Could you check a few things on this model? Use its own coordinates, in mm. A direction names the side the tool comes from. Give positions to 0.01 mm unless a question says otherwise; leave off trailing zeros. Loops run counter-clockwise (first coordinate to the right, second up) from the corner with the lowest first, then second, coordinate; pieces in that order, holes last. Notation, with made-up numbers: (32.25, 50.5) -> (47.25, 50.5) arc R17 ccw to (47.25, 75.5) -> close; hole circle Ø4 at (7.5, 70.5). An arc over 180 degrees is marked (long way). Put each result on its own line as item: value.
```python
from build123d import *

# Parameters (mm, degrees)
SKETCH1_R             = 25
BOSS_EXTRUDE1_DEPTH   = 12.38
BOSS_EXTRUDE4_START   = -5.38
SKETCH9_R             = 25
SKETCH9_R_2           = 9.525
BOSS_EXTRUDE4_DEPTH   = 5.38
SKETCH4_OUTSIDE_W     = 66.358
SKETCH4_OUTSIDE_H     = 66.358
SKETCH4_OUTSIDE_R     = 22
TREAD_CLEARANCE_DEPTH = 38.460170849
CUT_EXTRUDE2_START    = 1
SKETCH5_OUTSIDE_W     = 58.688
SKETCH5_OUTSIDE_H     = 58.688
SKETCH5_OUTSIDE_R     = 21.7
CUT_EXTRUDE2_DEPTH    = 10.38
CUT_EXTRUDE3_DEPTH    = 10.38
CIRPATTERN4_COUNT     = 18


with BuildPart() as part:
    # Sketch1 → Boss-Extrude1 (new body)
    with BuildSketch(Plane.XY):
        with Locations(Location((0, 0, 0), (0, 0, 90))):
            Circle(SKETCH1_R)
        with BuildLine():
            Line((9.525, -7.110786438), (9.525, 7.110786438))
            ThreePointArc((9.525, 7.110786438), (9.448879533, 7.49346987), (9.232106781, 7.817893219))
            Line((9.232106781, 7.817893219), (7.817893219, 9.232106781))
            ThreePointArc((7.817893219, 9.232106781), (7.49346987, 9.448879533), (7.110786438, 9.525))
            Line((7.110786438, 9.525), (-7.110786438, 9.525))
            ThreePointArc((-7.110786438, 9.525), (-7.49346987, 9.448879533), (-7.817893219, 9.232106781))
            Line((-7.817893219, 9.232106781), (-9.232106781, 7.817893219))
            ThreePointArc((-9.232106781, 7.817893219), (-9.448879533, 7.49346987), (-9.525, 7.110786438))
            Line((-9.525, 7.110786438), (-9.525, -7.110786438))
            ThreePointArc((-9.525, -7.110786438), (-9.448879533, -7.49346987), (-9.232106781, -7.817893219))
            Line((-9.232106781, -7.817893219), (-7.817893219, -9.232106781))
            ThreePointArc((-7.817893219, -9.232106781), (-7.49346987, -9.448879533), (-7.110786438, -9.525))
            Line((-7.110786438, -9.525), (7.110786438, -9.525))
            ThreePointArc((7.110786438, -9.525), (7.49346987, -9.448879533), (7.817893219, -9.232106781))
            Line((7.817893219, -9.232106781), (9.232106781, -7.817893219))
            ThreePointArc((9.232106781, -7.817893219), (9.448879533, -7.49346987), (9.525, -7.110786438))
        make_face(mode=Mode.SUBTRACT)
    extrude(amount=BOSS_EXTRUDE1_DEPTH)

    # Sketch9 → Boss-Extrude4 (add)
    with BuildSketch(Plane.XY.offset(12.38).offset(BOSS_EXTRUDE4_START)):
        with Locations(Location((0, 0, 0), (0, 0, 90))):
            Circle(SKETCH9_R)
        Circle(SKETCH9_R_2, mode=Mode.SUBTRACT)
    extrude(amount=BOSS_EXTRUDE4_DEPTH)

    # Sketch4 outside → Tread Clearance (cut, through all)
    with BuildSketch(Plane.XY.offset(12.38)):
        Rectangle(SKETCH4_OUTSIDE_W, SKETCH4_OUTSIDE_H)
        Circle(SKETCH4_OUTSIDE_R, mode=Mode.SUBTRACT)
    extrude(amount=-TREAD_CLEARANCE_DEPTH, mode=Mode.SUBTRACT)

    # Sketch5 outside → Cut-Extrude2 (cut)
    with BuildSketch(Plane.XY.offset(CUT_EXTRUDE2_START)):
        Rectangle(SKETCH5_OUTSIDE_W, SKETCH5_OUTSIDE_H)
        with Locations(Location((0, 0, 0), (0, 0, 90))):
            Circle(SKETCH5_OUTSIDE_R, mode=Mode.SUBTRACT)
    extrude(amount=CUT_EXTRUDE2_DEPTH, mode=Mode.SUBTRACT)

    # Sketch6 → Cut-Extrude3 (cut)
    with BuildSketch(Plane.XY.offset(1)):
        with BuildLine():
            ThreePointArc((6.505756366, 20.361958768), (6.446827822, 19.666593295), (6.273572546, 18.99058418))
            ThreePointArc((6.273572546, 18.99058418), (6.465736016, 18.325211027), (7.157089189, 18.284235134))
            ThreePointArc((7.157089189, 18.284235134), (8.371042068, 18.936944495), (9.657089189, 19.432720561))
            ThreePointArc((9.657089189, 19.432720561), (8.132554572, 20.118438213), (6.559758729, 20.684766506))
            ThreePointArc((6.559758729, 20.684766506), (6.519461312, 20.525586959), (6.505756366, 20.361958768))
        make_face()
    cut_extrude3 = extrude(amount=CUT_EXTRUDE3_DEPTH, mode=Mode.SUBTRACT)

    # CirPattern4: Cut-Extrude3 ×18 about axis
    cirpattern4_axis = Axis((0, 0, 0), (0, 0, 1))
    for i in range(1, CIRPATTERN4_COUNT):
        add(cut_extrude3.rotate(cirpattern4_axis, i * 360 / CIRPATTERN4_COUNT), mode=Mode.SUBTRACT)


solid = part.part
```
1. I'm going to push flat-ended pins straight in: pin 1 (5 mm diameter, centred on y = 13, z = 1.5, fed in from -X); pin 2 (2 mm diameter, centred on x = -3.5, z = 10.5, fed in from -Y); pin 3 (2 mm diameter, centred on y = -0.5, z = 7, fed in from -X). Where does each tip first touch, or does it pass through?
Recorded:
pin 1: stops at x = -19.31
pin 2: stops at y = -21.79
pin 3: stops at x = -21.7
2. If we section it at A-A (x = -4): List the corners of the cut face in (y, z) for me (3 decimals), then the cut area to 3 significant figures.
Recorded:
outline: (-21.633, 0) -> (-9.525, 0) -> (-9.525, 7) -> (-8.644, 7) -> (-8.644, 12.38) -> (-21.633, 12.38) -> (-21.633, 11.38) -> (-21.328, 11.38) -> (-21.328, 1) -> (-21.633, 1) -> close; (8.644, 7) -> (9.525, 7) -> (9.525, 0) -> (21.633, 0) -> (21.633, 1) -> (21.328, 1) -> (21.328, 11.38) -> (21.633, 11.38) -> (21.633, 12.38) -> (8.644, 12.38) -> close
area: 303 mm^2
3. I need wall thicknesses on line 1 (X direction, y = 0, z = 8.65) (3 decimals); line 2 (Y direction, x = 0, z = 9.55) (3 decimals); line 3 (X direction, y = -5, z = 8.75). Which ranges of each line are inside material? Lowest first, please.
Recorded:
line 1: x = -21.7 to -9.525, 9.525 to 21.7
line 2: y = -19.4 to -9.525, 9.525 to 19.4
line 3: x = -21.12 to -8.11, 8.11 to 20.13
4. Thinking about a two-plate mould opening in Z: for faces 5 (the face through (7, 7, 7)), 6 (the face through (18.57, 9.13, 6.12)), 7 (the face through (8.52, -8.53, 3.45)), which applies, pulls with the +Z half, pulls with the -Z half, needs draft (parallel to the pull), parting line crosses it, or undercut?
Recorded:
face 5: pulls with the -Z half
face 6: undercut
face 7: needs draft
5. For faces 1 (the face through (-11.5, -18.4, 6.1)), 2 (the face through (20.57, 2.23, 6.12)), 3 (the face through (20.65, 6.67, 6.12)), 4 (the face through (-19.105, -3.573, 6.117)), which set-ups out of +Z, -Z, +X, -X, +Y, -Y let a thin tool reach every point of the face, with its end or its side?
Recorded:
face 1: -X, -Y
face 2: +X
face 3: +X, +Y
face 4: -X
